Could you check a few things on this model? Use its own coordinates, in mm. Face numbers are marked on the shaded views. A direction names the side the tool comes from. Round coordinates to 2 decimals unless told otherwise and drop trailing zeros. Loops run counter-clockwise (first coordinate to the right, second up) from the corner with the lowest first, then second, coordinate; pieces in that order, holes last. Notation, with made-up numbers: (37.5, 63) -> (46.5, 63) arc R8 cw to (46.5, 76) -> close; hole circle Ø3 at (79.25, -3.75). An arc over 180 degrees is marked (long way). One line per item, written item: value.
```python
from build123d import *

# Parameters (mm, degrees)
F0_W     = 45.72
F0_H     = 49.53
F1_DEPTH = 5.842
F2_R     = 2.54
F3_DEPTH = 25.4
F4_R     = 3.81
F5_DEPTH = 4.064
F6_R     = 2.54
F7_DEPTH = 25.4
F8_R     = 5.08


# Not quite as in the source:
# - a feature names something its author has since deleted; it is built from what else it names


with BuildPart() as f1:
    # F0 (on Top) → F1 (new body)
    with BuildSketch(Plane.XY):
        Rectangle(F0_W, F0_H)
    extrude(amount=F1_DEPTH)

    # F2 (on face) → F3 (cut)
    with BuildSketch(Plane.XY.offset(5.842)):
        with Locations((-19.8755, 0)):
            Circle(F2_R)
        with Locations((19.8755, 0)):
            Circle(F2_R)
    extrude(amount=-F3_DEPTH, mode=Mode.SUBTRACT)

    # F4 (on face) → F5 (cut)
    with BuildSketch(Plane.XY.offset(5.842)):
        with Locations((0, 20.701)):
            Circle(F4_R)
        with Locations((0, -20.701)):
            Circle(F4_R)
    extrude(amount=-F5_DEPTH, mode=Mode.SUBTRACT)

    # F6 (on face) → F7 (cut)
    with BuildSketch(Plane.XY.offset(5.842)):
        with Locations((0, 20.701)):
            Circle(F6_R)
        with Locations((0, -20.701)):
            Circle(F6_R)
    extrude(amount=-F7_DEPTH, mode=Mode.SUBTRACT)

    # F8
    f8_edges = [f1.edges().sort_by_distance(p)[0] for p in [
        (-22.86, 24.765, 2.921),
        (-22.86, -24.765, 2.921),
        (22.86, -24.765, 2.921),
        (22.86, 24.765, 2.921),
    ]]
    fillet(f8_edges, radius=F8_R)


solid = f1.part
```
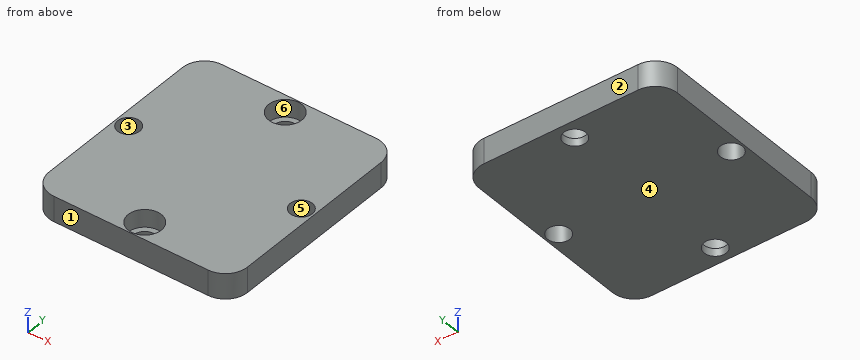
(1) Imagine slicing it at C-C on z = 4.85. Write out the boundary of the cut face in (x, y) (1 decimal), then the cut area to 3 significant figures.
Results below:
outline: (-22.9, -19.7) arc R5.1 ccw to (-17.8, -24.8) -> (17.8, -24.8) arc R5.1 ccw to (22.9, -19.7) -> (22.9, 19.7) arc R5.1 ccw to (17.8, 24.8) -> (-17.8, 24.8) arc R5.1 ccw to (-22.9, 19.7) -> close; hole circle Ø5.1 at (-19.9, 0); hole circle Ø7.6 at (0, -20.7); hole circle Ø7.6 at (0, 20.7); hole circle Ø5.1 at (19.9, 0)
area: 2,110 mm²
(2) For pin 1 Ø4 at (x, y) = (1.5, 20.5) entering from +Z; pin 2 Ø4.5 at (x, y) = (0, -20.701) entering from -Z, each with a flat end and sliding along its axis, tell me the tip position at first contact or that it passes through.
Results below:
pin 1: stops at z = 1.78
pin 2: passes through
(3) Please list where these lines run through material, in increasing order: L1, parallel to Y at x = 0, z = 1.35 (3 decimals); L2, parallel to Y at x = 0, z = 3.15 (3 decimals); L3, parallel to X at y = 1, z = 5.5.
Results below:
L1: y = -24.765 to -23.241, -18.161 to 18.161, 23.241 to 24.765
L2: y = -24.765 to -24.511, -16.891 to 16.891, 24.511 to 24.765
L3: x = -22.86 to -22.21, -17.54 to 17.54, 22.21 to 22.86
(4) On a 3-axis mill with a long thin cutter (end or side, diameter ignored), from which of +Z, -Z, +X, -X, +Y, -Y can I reach the whole of each face in a straight line? I mean the marked faces 5 and 6. Say none if no direction works.
Results below:
face 5: +Z, -Z
face 6: +Z
(5) Imagine slicing it at A-A on x = 0. Write out the boundary of the cut face in (y, z) (3 decimals).
Results below:
outline: (-24.765, 0) -> (-23.241, 0) -> (-23.241, 1.778) -> (-24.511, 1.778) -> (-24.511, 5.842) -> (-24.765, 5.842) -> close; (-18.161, 0) -> (18.161, 0) -> (18.161, 1.778) -> (16.891, 1.778) -> (16.891, 5.842) -> (-16.891, 5.842) -> (-16.891, 1.778) -> (-18.161, 1.778) -> close; (23.241, 0) -> (24.765, 0) -> (24.765, 5.842) -> (24.511, 5.842) -> (24.511, 1.778) -> (23.241, 1.778) -> close
(6) We'd pull the mould along Y, two halves only. Please class the marked faces 1, 2, 3 and 4: +Y half, -Y half, draft (parallel to the pull), parting line (faces both ways), or undercut.
Results below:
face 1: -Y half
face 2: +Y half
face 3: undercut
face 4: draft
(7) Imagine slicing it at B-B on y = 0. Write out the boundary of the cut face in (x, z), then the cut area to 3 significant figures.
Results below:
outline: (-22.86, 0) -> (-22.42, 0) -> (-22.42, 5.84) -> (-22.86, 5.84) -> close; (-17.34, 0) -> (17.34, 0) -> (17.34, 5.84) -> (-17.34, 5.84) -> close; (22.42, 0) -> (22.86, 0) -> (22.86, 5.84) -> (22.42, 5.84) -> close
area: 208 mm²
